Could you check a few things on this model? Use its own coordinates, in mm. A direction names the side the tool comes from. Coordinates: 2 decimals unless noted, no trailing zeros. Write each loop counter-clockwise with the first axis right and the second up, starting at its lowest first coordinate (ties: lowest second). Pieces come first, ordered by that corner, then holes.
Item 1: If I drill on probe 1 along Z at (x, y) = (-8.05, 0); probe 2 along X at (y, z) = (9, -10), over which ranges is the centre line in solid material (lowest first)?
Item 2: For P1, Ø12, axis at x = -15, z = 4.5, coming from the +Y side; P2, Ø8, axis at x = -8.5, y = 6.5, coming from the -Z side; P3, Ø11, axis at y = 4, z = -0.5, coming from the +X side, each with a flat end and sliding along its axis, tell me the tip position at first contact or that it passes through.
Item 3: I want a section at A-A on x = 7.5. Please give me the cut outline in (y, z).
Item 4: Which directions (+Z, -Z, +X, -X, +Y, -Y) give clear straight access to the entire face, cutting with the end or side of a thin tool? Please do faces 1 (the cylindrical face through (0.04, 0.53, 11.99)), 2 (the cylindrical face through (7.4, -12, 2.7)), 3 (the cylindrical face through (-2.3, 3.27, -10.4)).
Item 5: Thinking about a two-plate mould opening in Z: for faces 4 (the conical face through (3, -11, 2)), 5 (the flat face through (-17.75, 0, 0)), 6 (the cylindrical face through (-5.411, -0.668, 15.185)), which applies, +Z half, -Z half, draft (parallel to the pull), parting line (faces both ways), or undercut?
Item 6: I want a section at B-B on x = -5.75. Please give me the cut outline in (y, z), then the cut area to 3 significant figures.
Autodesk Inventor part; units mm, degrees
ref_plane "YZ Plane" through (0, 0, 0) normal (1, 0, 0) x (0, 1, 0)
ref_plane "XZ Plane" through (0, 0, 0) normal (0, 1, 0) x (-1, 0, 0)
ref_plane "XY Plane" through (0, 0, 0) normal (0, 0, 1) x (1, 0, 0)
sketch "Sketch1" plane through (0, 0, 0) normal (0, 1, 0) x (-1, 0, 0)
  line L0 (0, 0) -> (10.1, 0) construction
  line L1 (10.1, 0) -> (10.1, -10.9) construction
  line L2 (10.1, -10.9) -> (0, -10.9) construction
  line L3 (0, -10.9) -> (0, 0) construction
  line L4 (10.1, 0) -> (4.6, 0) construction
  line L5 (4.6, 0) -> (4.6, -12.3) construction
  line L6 (4.6, -12.3) -> (10.1, -12.3) construction
  line L7 (10.1, -12.3) -> (10.1, 0) construction
  line L8 (4.6, -10.9) -> (2.6, -10.9) construction
  line L9 (2.6, -10.9) -> (4.6, -12.3) construction
  line L10 (0, 0) -> (17.75, 0) construction
  line L11 (17.75, 0) -> (17.75, -6) construction
  line L12 (17.75, -6) -> (0, -6) construction
  line L13 (0, -6) -> (0, 0) construction
  line L14 (10.1, 0) -> (8.5, 0) construction
  line L15 (8.5, 0) -> (8.5, -15.2) construction
  line L16 (8.5, -15.2) -> (10.1, -15.2) construction
  line L17 (10.1, -15.2) -> (10.1, 0) construction
  line L18 (8.5, 0) -> (6.2, 0) construction
  line L19 (6.2, 0) -> (6.2, -13.2) construction
  line L20 (6.2, -13.2) -> (8.5, -13.2) construction
  line L21 (8.5, -13.2) -> (8.5, 0) construction
  line L22 (0, 0) -> (0, -12) construction
  line L23 (0, -12) -> (2.6, -12) construction
  line L24 (6.2, 0) -> (4.6, 0) construction
  line L25 (4.6, 0) -> (4.6, -15.2) construction
  line L26 (4.6, -15.2) -> (6.2, -15.2) construction
  line L27 (6.2, -15.2) -> (6.2, 0) construction
  line L28 (4.6, -15.2) -> (4.6, -13.3) construction
  line L29 (4.6, -13.3) -> (2.6, -12) construction
  line L30 (0, 0) -> (-10.1, 0) construction
  line L31 (-10.1, 0) -> (-10.1, -10.9) construction
  line L32 (-10.1, -10.9) -> (0, -10.9) construction
  line L33 (-10.1, 0) -> (-4.6, 0) construction
  line L34 (-4.6, 0) -> (-4.6, -12.3) construction
  line L35 (-4.6, -12.3) -> (-10.1, -12.3) construction
  line L36 (-10.1, -12.3) -> (-10.1, 0) construction
  line L37 (-4.6, -10.9) -> (-2.6, -10.9) construction
  line L38 (-2.6, -10.9) -> (-4.6, -12.3) construction
  line L39 (-10.1, 0) -> (-8.5, 0) construction
  line L40 (-8.5, 0) -> (-8.5, -15.2) construction
  line L41 (-8.5, -15.2) -> (-10.1, -15.2) construction
  line L42 (-10.1, -15.2) -> (-10.1, 0) construction
  line L43 (-8.5, 0) -> (-6.2, 0) construction
  line L44 (-6.2, 0) -> (-6.2, -13.2) construction
  line L45 (-6.2, -13.2) -> (-8.5, -13.2) construction
  line L46 (-8.5, -13.2) -> (-8.5, 0) construction
  line L47 (0, -12) -> (-2.6, -12) construction
  line L48 (-6.2, 0) -> (-4.6, 0) construction
  line L49 (-4.6, 0) -> (-4.6, -15.2) construction
  line L50 (-4.6, -15.2) -> (-6.2, -15.2) construction
  line L51 (-6.2, -15.2) -> (-6.2, 0) construction
  line L52 (-4.6, -15.2) -> (-4.6, -13.3) construction
  line L53 (-4.6, -13.3) -> (-2.6, -12) construction
  line L54 (0, 0) -> (-2, 0) construction
  line L55 (-2, 0) -> (-2, -10.9) construction
  line L56 (-2, -10.9) -> (0, -10.9) construction
  line L57 (0, -10.9) -> (0, 0) construction
  line L58 (0, 0) -> (2, 0) construction
  line L59 (2, 0) -> (2, -10.9) construction
  line L60 (2, -10.9) -> (0, -10.9) construction
  line L61 (0, -10.9) -> (0, 0) construction
  line L62 (0, -6) -> (-8.5, -6) construction
  line L63 (-8.5, -6) -> (-8.5, 0) construction
  line L64 (-8.5, 0) -> (0, 0) construction
  line L65 (0, 0) -> (0, -6) construction
  line L66 (10.1, -12.3) -> (8.5, -12.3) construction
  line L67 (8.5, -12.3) -> (6.2, -12.3) construction
  line L68 (4.6, -12.3) -> (4.6, -13.3) construction
  line L69 (2.6, -12) -> (2.6, -10.9) construction
  line L70 (-2.6, -10.9) -> (-4.6, -12.3) construction
  line L71 (-6.2, -12.3) -> (-8.5, -12.3) construction
  line L72 (-10.1, -12.3) -> (-10.1, -15.2) construction
  line L73 (-8.5, -15.2) -> (-8.5, -13.2) construction
  line L74 (-6.2, -13.2) -> (-6.2, -15.2) construction
  line L75 (10.1, -12.3) -> (4.6, -12.3) construction
  line L76 (2.6, -10.9) -> (2, -10.9) construction
  line L77 (2, -6) -> (17.75, -6) construction
  line L78 (17.75, 0) -> (-8.5, 0) construction
  line L79 (-8.5, -6) -> (-2, -6) construction
  line L80 (-2, -10.9) -> (-2.6, -10.9) construction
  line L81 (-4.6, -12.3) -> (-10.1, -12.3) construction
  line L82 (-10.1, -15.2) -> (-8.5, -15.2) construction
  line L83 (17.75, 0) -> (17.75, -6)
  line L84 (2, -6) -> (2, -10.9)
  line L85 (2.6, -10.9) -> (4.6, -12.3)
  line L86 (10.1, -12.3) -> (10.1, -15.2)
  line L87 (8.5, -15.2) -> (8.5, -13.2)
  line L88 (6.2, -13.2) -> (6.2, -15.2)
  line L89 (4.6, -15.2) -> (4.6, -13.3)
  line L90 (2.6, -12) -> (-2.6, -12)
  line L91 (-4.6, -13.3) -> (-4.6, -15.2)
  line L92 (-6.2, -15.2) -> (-6.2, -13.2)
  line L93 (-8.5, -13.2) -> (-8.5, -15.2)
  line L94 (-10.1, -15.2) -> (-10.1, -12.3)
  line L95 (-6.2, -13.2) -> (-8.5, -13.2)
  line L96 (-2.6, -12) -> (-4.6, -13.3)
  line L97 (-4.6, -12.3) -> (-10.1, -12.3)
  line L98 (4.6, -13.3) -> (2.6, -12)
  line L99 (4.6, -15.2) -> (6.2, -15.2)
  line L100 (-4.6, -12.3) -> (-2.6, -10.9)
  line L101 (-2, -10.9) -> (-2.6, -10.9)
  line L102 (-2, -6) -> (-2, -10.9)
  line L103 (8.5, -13.2) -> (6.2, -13.2)
  line L104 (8.5, -15.2) -> (10.1, -15.2)
  line L105 (10.1, -12.3) -> (4.6, -12.3)
  line L106 (17.75, -6) -> (2, -6)
  line L107 (17.75, 0) -> (-8.5, 0)
  line L108 (-8.5, -6) -> (-8.5, 0)
  line L109 (-8.5, -6) -> (-2, -6)
  line L110 (-4.6, -15.2) -> (-6.2, -15.2)
  line L111 (-8.5, -15.2) -> (-10.1, -15.2)
  line L112 (-2, -6) -> (-8.5, -6)
  line L113 (-8.5, -6) -> (-8.5, -7)
  line L114 (-8.5, -7) -> (-2, -7)
  line L115 (-2, -7) -> (-2, -6)
  line L116 (2, -6) -> (17.75, -6)
  line L117 (17.75, -6) -> (17.75, -7)
  line L118 (17.75, -7) -> (2, -7)
  line L119 (2, -7) -> (2, -6)
  line L120 (2.6, -10.9) -> (2, -10.9)
  dimension "d0" = 10.1
  dimension "d1" = 10.9
  dimension "d2" = 5.5
  dimension "d3" = 12.3
  dimension "d4" = 2
  dimension "d5" = 17.75
  dimension "d6" = 6
  dimension "d7" = 1.6
  dimension "d8" = 15.2
  dimension "d9" = 2.3
  dimension "d10" = 13.2
  dimension "d12" = 12
  dimension "d13" = 2.6
  dimension "d15" = 15.2
  dimension "d16" = 1.9
  dimension "d17" = 2
  dimension "d18" = 2
  dimension "d19" = 1
  dimension "d20" = 1
revolve "Revolution1" add sketch "Sketch1" angle 360 about axis through (0, 0, 0) along (-1, 0, 0) contours L83 L106 L84 L120 L85 L105 L86 L104 L87 L103 L88 L99 L89 L98 L90 L96 L91 L110 L92 L95 L93 L111 L94 L97 L100 L101 L102 L109 L108 L107
sketch "Sketch2" plane through (0, 0, 0) normal (1, 0, 0) x (0, 1, 0)
  line L0 (0, 0) -> (0, 12)
  circle A0 centre (0, 0) radius 12
  line L1 (0, 12) -> (0, 15.2)
  circle A1 centre (0, 0) radius 15.2
  line L2 (-1.5, 15.2) -> (1.5, 15.2)
  line L3 (-1.5, 15.2) -> (0, 15.2)
  line L4 (0, 15.2) -> (0, 0)
  line L5 (0, 0) -> (-1.5, 0)
  line L6 (-1.5, 0) -> (-1.5, 15.2)
  line L7 (0, 0) -> (1.5, 0)
  line L8 (1.5, 0) -> (1.5, 15.2)
  line L9 (1.5, 15.2) -> (0, 15.2)
  line L10 (0, 15.2) -> (0, 0)
  line L11 (0, 0) -> (-12, 0)
  line L12 (-12, 0) -> (-15.2, 0)
  line L13 (-15.2, -1.5) -> (-15.2, 1.5)
  line L14 (-15.2, -1.5) -> (-15.2, 0)
  line L15 (-15.2, 0) -> (0, 0)
  line L16 (0, 0) -> (0, -1.5)
  line L17 (0, -1.5) -> (-15.2, -1.5)
  line L18 (0, 0) -> (0, 1.5)
  line L19 (0, 1.5) -> (-15.2, 1.5)
  line L20 (-15.2, 1.5) -> (-15.2, 0)
  line L21 (-15.2, 0) -> (0, 0)
  line L22 (0, 0) -> (0, -12)
  line L23 (0, -12) -> (0, -15.2)
  line L24 (1.5, -15.2) -> (-1.5, -15.2)
  line L25 (1.5, -15.2) -> (0, -15.2)
  line L26 (0, -15.2) -> (0, 0)
  line L27 (0, 0) -> (1.5, 0)
  line L28 (1.5, 0) -> (1.5, -15.2)
  line L29 (0, 0) -> (-1.5, 0)
  line L30 (-1.5, 0) -> (-1.5, -15.2)
  line L31 (-1.5, -15.2) -> (0, -15.2)
  line L32 (0, -15.2) -> (0, 0)
  line L33 (0, 0) -> (12, 0)
  line L34 (12, 0) -> (15.2, 0)
  line L35 (15.2, 1.5) -> (15.2, -1.5)
  line L36 (15.2, 1.5) -> (15.2, 0)
  line L37 (15.2, 0) -> (0, 0)
  line L38 (0, 0) -> (0, 1.5)
  line L39 (0, 1.5) -> (15.2, 1.5)
  line L40 (0, 0) -> (0, -1.5)
  line L41 (0, -1.5) -> (15.2, -1.5)
  line L42 (15.2, -1.5) -> (15.2, 0)
  line L43 (15.2, 0) -> (0, 0)
  dimension "d22" = 3
  dimension "d25" = 360
properties part number "Wheel Rim"
Response values:
1. probe 1: z = -13.2 to -12.3, -6 to 6, 12.3 to 13.2
1. probe 2: x = -10.1 to -8.5, -6.2 to -4.6, 4.6 to 6.2, 8.5 to 10.1
2. P1: stops at y = 15.16
2. P2: stops at z = -14.99
2. P3: stops at x = 8.5
3. outline: circle Ø26.4 at (0, 0); circle Ø12 at (0, 0); hole circle Ø24.6 at (0, 0)
4. face 1: none
4. face 2: +X
4. face 3: -X
5. face 4: undercut
5. face 5: draft
5. face 6: parting line
6. outline: circle Ø30.4 at (0, 0); circle Ø12 at (0, 0); hole circle Ø24.6 at (0, 0)
6. area: 364 mm2
